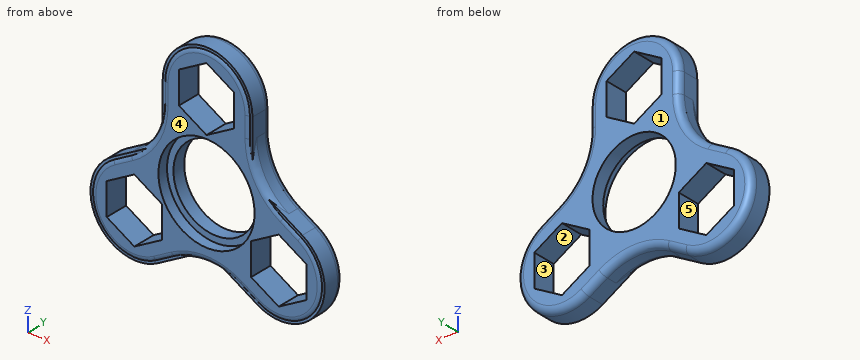
from build123d import *

# Parameters (mm, degrees)
F0_R     = 13
F1_DEPTH = 3.6
F2_R     = 20
F3_R     = 2
F4_R     = 2
F5_DEPTH = 3.2
F6_R     = 15
F7_DEPTH = 3.2


# Not quite as in the source:
# - a feature names something its author has since deleted; it is built from what else it names


with BuildPart() as f1:
    # F0 (on Front) → F1 (new body, symmetric)
    with BuildSketch(Plane.XZ):
        with BuildLine():
            Line((14, 8.0829037687), (14, 26))
            ThreePointArc((14, 26), (0, 40), (-14, 26))
            Line((-14, 26), (-14, 8.0829037687))
            Line((-14, 8.0829037687), (-29.5166604984, -0.875644347))
            ThreePointArc((-29.5166604984, -0.875644347), (-34.6410161514, -20), (-15.5166604984, -25.124355653))
            Line((-15.5166604984, -25.124355653), (0, -16.1658075373))
            Line((0, -16.1658075373), (15.5166604984, -25.124355653))
            ThreePointArc((15.5166604984, -25.124355653), (34.6410161514, -20), (29.5166604984, -0.875644347))
            Line((29.5166604984, -0.875644347), (14, 8.0829037687))
        make_face()
        Polygon((-22.5166604984, -22.9304246301), (-31.1166604984, -17.965212315), (-31.1166604984, -8.034787685), (-22.5166604984, -3.0695753699), (-13.9166604984, -8.034787685), (-13.9166604984, -17.965212315), align=None, mode=Mode.SUBTRACT)
        Polygon((31.1166604984, -8.034787685), (31.1166604984, -17.965212315), (22.5166604984, -22.9304246301), (13.9166604984, -17.965212315), (13.9166604984, -8.034787685), (22.5166604984, -3.0695753699), align=None, mode=Mode.SUBTRACT)
        Circle(F0_R, mode=Mode.SUBTRACT)
        Polygon((0, 35.9304246301), (8.6, 30.965212315), (8.6, 21.034787685), (0, 16.0695753699), (-8.6, 21.034787685), (-8.6, 30.965212315), align=None, mode=Mode.SUBTRACT)
    extrude(amount=F1_DEPTH, both=True)

    # F2
    f2_edges = [f1.edges().sort_by_distance(p)[0] for p in [
        (0, 0, -16.165808),
        (14, 0, 8.082904),
        (-14, 0, 8.082904),
    ]]
    fillet(f2_edges, radius=F2_R)

    # F3
    f3_edges = [f1.edges().sort_by_distance(p)[0] for p in [
        (-14, -3.6, 22.814955),
    ]]
    fillet(f3_edges, radius=F3_R)

    # F4
    f4_edges = [f1.edges().sort_by_distance(p)[0] for p in [
        (0, 3.6, 40),
        (26.75833, 3.6, 0.716878),
        (16.679492, 3.6, 9.629909),
        (34.641016, 3.6, -20),
        (14, 3.6, 22.814955),
        (12.75833, 3.6, -23.531833),
        (0, 3.6, -19.259818),
        (-14, 3.6, 22.814955),
        (-12.75833, 3.6, -23.531833),
        (-16.679492, 3.6, 9.629909),
        (-34.641016, 3.6, -20),
        (-26.75833, 3.6, 0.716878),
    ]]
    fillet(f4_edges, radius=F4_R)

    # F0 (on Front) → F5 (join)
    with BuildSketch(Plane.XZ):
        with BuildLine():
            Line((14, 8.0829037687), (14, 26))
            ThreePointArc((14, 26), (0, 40), (-14, 26))
            Line((-14, 26), (-14, 8.0829037687))
            Line((-14, 8.0829037687), (-29.5166604984, -0.875644347))
            ThreePointArc((-29.5166604984, -0.875644347), (-34.6410161514, -20), (-15.5166604984, -25.124355653))
            Line((-15.5166604984, -25.124355653), (0, -16.1658075373))
            Line((0, -16.1658075373), (15.5166604984, -25.124355653))
            ThreePointArc((15.5166604984, -25.124355653), (34.6410161514, -20), (29.5166604984, -0.875644347))
            Line((29.5166604984, -0.875644347), (14, 8.0829037687))
        make_face()
        Polygon((-22.5166604984, -22.9304246301), (-31.1166604984, -17.965212315), (-31.1166604984, -8.034787685), (-22.5166604984, -3.0695753699), (-13.9166604984, -8.034787685), (-13.9166604984, -17.965212315), align=None, mode=Mode.SUBTRACT)
        Polygon((31.1166604984, -8.034787685), (31.1166604984, -17.965212315), (22.5166604984, -22.9304246301), (13.9166604984, -17.965212315), (13.9166604984, -8.034787685), (22.5166604984, -3.0695753699), align=None, mode=Mode.SUBTRACT)
        Circle(F0_R, mode=Mode.SUBTRACT)
        Polygon((0, 35.9304246301), (8.6, 30.965212315), (8.6, 21.034787685), (0, 16.0695753699), (-8.6, 21.034787685), (-8.6, 30.965212315), align=None, mode=Mode.SUBTRACT)
    extrude(amount=F5_DEPTH)

    # F6 (on face) → F7 (cut)
    with BuildSketch(Plane.XZ.offset(3.6)):
        Circle(F6_R)
    extrude(amount=-F7_DEPTH, mode=Mode.SUBTRACT)


solid = f1.part
Input: part model. Units: mm. Frame: model coordinates. Face numbers are marked on the shaded views. A direction names the side the tool comes from. Coordinates: 2 decimals unless noted, no trailing zeros. Write each loop counter-clockwise with the first axis right and the second up, starting at its lowest first coordinate (ties: lowest second). Pieces come first, ordered by that corner, then holes. Notation, with made-up numbers: M 66,69 L 86,69 A16 ccw 86,83 Z; hole C 43.25,81.25 d7. An arc over 180 degrees is marked long. Answer as a JSON object with one key per item and string values. Group by question number.
(1) Ray query, line 1 along Z through (x, y) = (0, -1.2); line 2 along Z through (x, y) = (0, 1.95); line 3 along X through (y, z) = (-2.5, -16). Return the intervals inside material, ascending. Write a range as [from, to].
(2) Section A-A on z = 22. Output: boundary loops of the cut face in (x, y).
(3) Section B-B on y = 0.5. Give the number of separate pieces and of enclosed holes in the cut face, plus the area to 3 significant figures.
(4) Mould query, pull axis X, two halves, no side actions, for the marked faces 3, 4 and 5. Classes: pulls with the +X half, pulls with the -X half, needs draft (parallel to the pull), parting line crosses it, or undercut.
(5) Contact query for flat-ended pins moving along their axis: P1, Ø2, axis at y = 1.5, z = -10, coming from the -X side; P2, Ø12, axis at x = 0, z = 4, coming from the -Y side; P3, Ø2, axis at x = 24.5, y = -0.5, coming from the -Z side; P4, Ø2, axis at y = -0.5, z = 27.5, coming from the -X side. Output: stop coordinate, or through.
(6) Set-up query: the marked faces 1 and 2. Return all of +Z, -Z, +X, -X, +Y, -Y with unobstructed straight access to the full face (end or side cutting, diameter ignored); none if empty.
Result set:
{
 "1": {"line 1": "z = [-19.26, -15], [15, 16.07], [35.93, 40]", "line 2": "z = [-19.23, -13], [13, 16.07], [35.93, 39.97]", "line 3": "x = [-36.19, -31.12], [-13.92, 13.92], [31.12, 36.19]"},
 "2": {"outline": "M -14,-3.2 L -13.2,-3.2 A2 ccw -12,-3.6 L -8.6,-3.6 L -8.6,3.6 L -12,3.6 A2 ccw -14,1.6 Z; M 8.6,-3.6 L 12,-3.6 A2 ccw 13.2,-3.2 L 14,-3.2 L 14,1.6 A2 ccw 12,3.6 L 8.6,3.6 Z"},
 "3": {"separate pieces": "1", "enclosed holes": "4", "area": "1,530 mm2"},
 "4": {"face 3": "undercut", "face 4": "needs draft", "face 5": "undercut"},
 "5": {"P1": "stops at x = -36.37", "P2": "passes through", "P3": "stops at z = -26.97", "P4": "stops at x = -13.99"},
 "6": {"face 1": "+Z, -Z, +X, -X, +Y", "face 2": "+Y, -Y"}
}
